The figure shows three views and two pictorial views of one solid part (mm, origin at its lowest corner). Answer the questions. A direction names the side the tool comes from. Round coordinates to 2 decimals unless told otherwise and drop trailing zeros. Order: outer loops, then holes, each group sorted by start corner. A loop starts at its lowest first (then second) coordinate and runs counter-clockwise, first axis right, second up. Notation, with made-up numbers: (16.5, 87.5) - (62.5, 87.5) arc R19 ccw to (62.5, 95.5) - close; hole circle Ø9 at (68, 89.25). An arc over 180 degrees is marked (long way). Answer in a Markdown table with one row per item.
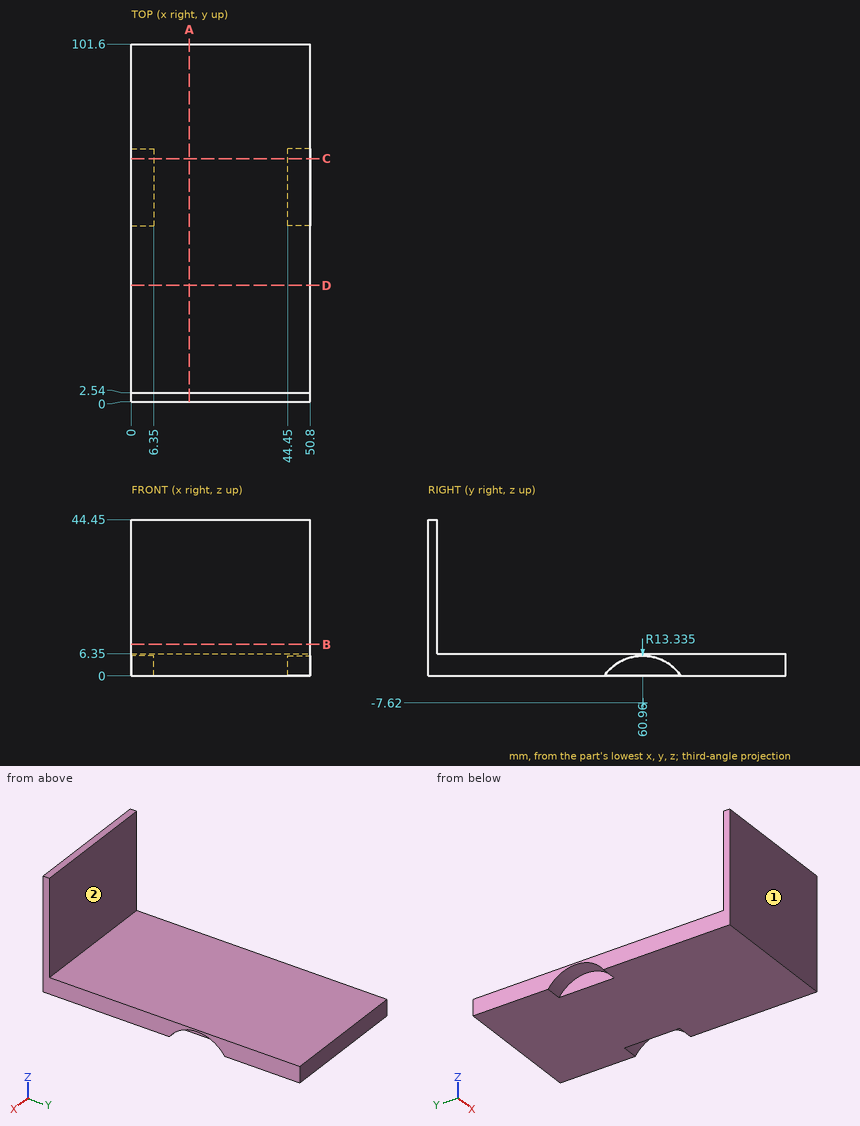
1) Each of these flat-tipped pins is pushed along its axis until it touches: pin 1 (1.5 mm diameter, centred on x = 9, y = 76.5, fed in from +Z); pin 2 (1.7 mm diameter, centred on y = 66, z = 3.5, fed in from -X); pin 3 (1 mm diameter, centred on x = 24.5, z = 37, fed in from +Y). Where does it stop, or does it pass through?
Filled in:
| item | result |
|---|---|
| pin 1 | stops at z = 6.35 |
| pin 2 | stops at x = 6.35 |
| pin 3 | stops at y = 2.54 |
2) Which of the six approach directions +Z, -Z, +X, -X, +Y, -Y give full straight-line access (tool end or side, diameter ignored) to the marked faces 1 and 2?
Filled in:
| item | result |
|---|---|
| face 1 | +Z, -Z, +X, -X, -Y |
| face 2 | +Z, +X, -X, +Y |
3) Find section B-B, the plane z = 9. Give the vertices of the cut face in (x, y), then the cut area to 3 significant figures.
Filled in:
| item | result |
|---|---|
| outline | (0, 0) - (50.8, 0) - (50.8, 2.54) - (0, 2.54) - close |
| area | 129 mm^2 |
4) Find section D-D, the plane y = 33. Give the vertices of the cut face in (x, z), then the cut area to 3 significant figures.
Filled in:
| item | result |
|---|---|
| outline | (0, 0) - (50.8, 0) - (50.8, 6.35) - (0, 6.35) - close |
| area | 323 mm^2 |
5) Find section C-C, the plane y = 69. Give the vertices of the cut face in (x, z), then the cut area to 3 significant figures.
Filled in:
| item | result |
|---|---|
| outline | (0, 3.02) - (6.35, 3.02) - (6.35, 0) - (44.45, 0) - (44.45, 3.02) - (50.8, 3.02) - (50.8, 6.35) - (0, 6.35) - close |
| area | 284 mm^2 |
6) Find the intervals of material crossed by probe 1 along Z at (x, y) = (33.5, 35); probe 2 along Y at (x, z) = (20, 41); probe 3 along Z at (x, y) = (45.5, 50.5), in increasing order. Write a range as from..to.
Filled in:
| item | result |
|---|---|
| probe 1 | z = 0..6.35 |
| probe 2 | y = 0..2.54 |
| probe 3 | z = 0.65..6.35 |
7) Find section A-A, the plane x = 16.5. Give the vertices of the cut face in (y, z).
Filled in:
| item | result |
|---|---|
| outline | (0, 0) - (101.6, 0) - (101.6, 6.35) - (2.54, 6.35) - (2.54, 44.45) - (0, 44.45) - close |
